Geometry check sheet. Reference: the model listing, model coordinates, mm. A direction names the side the tool comes from. Coordinates: 2 decimals unless noted, no trailing zeros. Order: outer loops, then holes, each group sorted by start corner. A loop starts at its lowest first (then second) coordinate and runs counter-clockwise, first axis right, second up. Notation, with made-up numbers: (23, 58.5) - (77, 58.5) arc R4 ccw to (77, 65.5) - close; hole circle Ø9 at (25, 61). An arc over 180 degrees is marked (long way). Put each result on its own line as item: value.
from build123d import *

# Parameters (mm, degrees)
SKETCH1_W                             = 152.4
SKETCH1_H                             = 203.2
BASE_DEPTH                            = 6.35
SKETCH2_W                             = 76.2
SKETCH2_H                             = 6.35
MOUNT_WALLS_DEPTH                     = 50.8
MOUNT_SUPPORT_DEPTH                   = 4.7625
F_24_0_152_DIAMETER_HOLE1_D           = 3.8608
F_24_0_152_DIAMETER_HOLE1_CSINK_D     = 5.1308
F_24_0_152_DIAMETER_HOLE1_CSINK_ANGLE = 90
SKETCH6_R                             = 8.89
SKETCH6_R_2                           = 1.55
CUT_EXTRUDE1_DEPTH                    = 149.785256326
SKETCH7_R                             = 10.16
SKETCH7_R_2                           = 1.55
CUT_EXTRUDE2_DEPTH                    = 6.35
CUT_EXTRUDE3_REACH                    = 138.783
SKETCH8_W                             = 38.1
SKETCH8_H                             = 101.6


with BuildPart() as part:
    # Sketch1 → base (new body)
    with BuildSketch(Plane.XY):
        Rectangle(SKETCH1_W, SKETCH1_H)
    extrude(amount=BASE_DEPTH)

    # Sketch2 → mount walls (add)
    with BuildSketch(Plane.XY.offset(6.35)):
        with Locations((38.1, -9.525)):
            Rectangle(SKETCH2_W, SKETCH2_H)
        with Locations((38.1, -60.325)):
            Rectangle(SKETCH2_W, SKETCH2_H)
    extrude(amount=MOUNT_WALLS_DEPTH)

    # Sketch3 → mount support (add)
    with BuildSketch(Plane(origin=(76.2, 0, 0), x_dir=(0, 0, -1), z_dir=(1, 0, 0))):
        Polygon((-6.35, -88.9), (-57.15, -63.5), (-6.35, -63.5), align=None)
        Polygon((-57.15, -6.35), (-6.35, 19.05), (-6.35, -6.35), align=None)
    mount_support = extrude(amount=-MOUNT_SUPPORT_DEPTH)

    # Mirror1: mount support across plane
    add(mount_support.mirror(Plane(origin=(38.1, 0, 0), x_dir=(0, 0, 1), z_dir=(1, 0, 0))))

    # #24 (0.152) Diameter Hole1 (through all)
    with Locations(Plane.XY.offset(6.35)):
        with Locations((-66.675, -92.075), (-66.675, 43.307), (-23.241, 43.307), (-23.241, -92.075), (-67.6275, 68.707), (-22.2885, 68.707)):
            CounterSinkHole(F_24_0_152_DIAMETER_HOLE1_D / 2, F_24_0_152_DIAMETER_HOLE1_CSINK_D / 2, counter_sink_angle=F_24_0_152_DIAMETER_HOLE1_CSINK_ANGLE)

    # Sketch6 → Cut-Extrude1 (cut, through all)
    with BuildSketch(Plane.XZ.offset(12.7)):
        with Locations((38.1, 38.1)):
            Circle(SKETCH6_R)
        with Locations((38.1, 50.62855)):
            Circle(SKETCH6_R_2)
        with Locations((38.1, 25.57145)):
            Circle(SKETCH6_R_2)
    extrude(amount=-CUT_EXTRUDE1_DEPTH, mode=Mode.SUBTRACT)

    # Sketch7 → Cut-Extrude2 (cut)
    with BuildSketch(Plane(origin=(0, -57.15, 0), x_dir=(1, 0, 0), z_dir=(0, 1, 0))):
        with Locations(Location((38.1, -38.1, 0), (0, 0, 180))):
            Circle(SKETCH7_R)
        with Locations(Location((24.2576, -46.091913366, 0), (0, 0, 180))):
            Circle(SKETCH7_R_2)
        with Locations(Location((38.1, -22.116173268, 0), (0, 0, 180))):
            Circle(SKETCH7_R_2)
        with Locations(Location((51.9424, -46.091913366, 0), (0, 0, 180))):
            Circle(SKETCH7_R_2)
    extrude(amount=-CUT_EXTRUDE2_DEPTH, mode=Mode.SUBTRACT)

    # Sketch8 → Cut-Extrude3 (cut, up to next)
    with BuildSketch(Plane.XY.offset(6.35), mode=Mode.PRIVATE) as cut_extrude3_sk1:
        Polygon((76.2, 42.338114892), (-35.744340046, 101.6), (76.2, 101.6), align=None)
    cut_extrude3_tool1 = extrude(cut_extrude3_sk1.sketch, amount=-CUT_EXTRUDE3_REACH, mode=Mode.PRIVATE) & part.part
    # Sketch8 → Cut-Extrude3 (cut, up to next)
    with BuildSketch(Plane.XY.offset(6.35), mode=Mode.PRIVATE) as cut_extrude3_sk2:
        with Locations((-44.31191896, -19.722477487)):
            Rectangle(SKETCH8_W, SKETCH8_H)
    cut_extrude3_tool2 = extrude(cut_extrude3_sk2.sketch, amount=-CUT_EXTRUDE3_REACH, mode=Mode.PRIVATE) & part.part
    add(cut_extrude3_tool1.solids().sort_by_distance((38.88522, 81.846038, 6.35))[0], mode=Mode.SUBTRACT)
    add(cut_extrude3_tool2.solids().sort_by_distance((-44.311919, -19.722477, 6.35))[0], mode=Mode.SUBTRACT)


solid = part.part
Q1. Thickness scan on L1, parallel to Z at x = 38, y = -60; L2, parallel to X at y = 5.5, z = 12.5; L3, parallel to Y at x = 43, z = 50.5. Record the ranges inside material, lowest first. Write a range as [from, to].
Answer block:
L1: z = [0, 20.57], [23.66, 27.94], [48.26, 57.15]
L2: x = [0, 4.76], [71.44, 76.2]
L3: y = [-63.5, -57.15], [-12.7, -6.35]
Q2. Section check B-B on y = -52. Record the boundary of the cut face in (x, z), then the cut area to 3 significant figures.
Answer block:
outline: (-76.2, 0) - (-63.36, 0) - (-63.36, 6.35) - (-76.2, 6.35) - close; (-25.26, 0) - (76.2, 0) - (76.2, 6.35) - (-25.26, 6.35) - close
area: 726 mm^2
Q3. Draft check along Y on faces 1 (the flat face through (-1, -101.6, 3)), 2 (the flat face through (-1, 1, 0)), 3 (the flat face through (29, -12.7, 31)), 4 (the flat face through (2.35, 6.17, 32.11)). Enter one of: pulls with the +Y half, pulls with the -Y half, needs draft (parallel to the pull), parting line crosses it, or undercut.
Answer block:
face 1: pulls with the -Y half
face 2: needs draft
face 3: undercut
face 4: pulls with the +Y half
Q4. Section check D-D on y = 8. Record the boundary of the cut face in (x, z), then the cut area to 3 significant figures.
Answer block:
outline: (-76.2, 0) - (-63.36, 0) - (-63.36, 6.35) - (-76.2, 6.35) - close; (-25.26, 0) - (76.2, 0) - (76.2, 28.45) - (71.44, 28.45) - (71.44, 6.35) - (4.76, 6.35) - (4.76, 28.45) - (0, 28.45) - (0, 6.35) - (-25.26, 6.35) - close
area: 936 mm^2
Q5. Depth check by flat-ended pin: pin 1 Ø3.5 at (x, z) = (24.26, 46.09) entering from -Y; pin 2 Ø4 at (x, z) = (38.1, 50.63) entering from +Y; pin 3 Ø10 at (x, y) = (10.5, -57) entering from +Z; pin 4 Ø6 at (x, y) = (-66.675, 43.307) entering from +Z. Enter the tip coordinate at first touch or a pass-through.
Answer block:
pin 1: stops at y = -63.5
pin 2: stops at y = -6.35
pin 3: stops at z = 57.15
pin 4: stops at z = 6.35
Q6. Section check C-C on z = 38.1. State how many separate pieces and enclosed holes the cut face has, then the cut area to 3 significant figures.
Answer block:
separate pieces: 4
enclosed holes: 0
area: 907 mm^2
Q7. Section check A-A on x = -50. Record the boundary of the cut face in (y, z).
Answer block:
outline: (-101.6, 0) - (-70.52, 0) - (-70.52, 6.35) - (-101.6, 6.35) - close; (31.08, 0) - (101.6, 0) - (101.6, 6.35) - (31.08, 6.35) - close
Q8. Access from +Z, -Z, +X, -X, +Y, -Y to the whole of each face (thin tool, end or side, straight path). Record for faces 5 (the cylindrical face through (33.412, -60.281, 29.086)), 6 (the flat face through (-45, 31.078, 3)), 7 (the flat face through (4.763, 1, 20)), 8 (the flat face through (38, -57.15, 26)).
Answer block:
face 5: -Y
face 6: +Z, -Z
face 7: +Z, +Y
face 8: +Z, +X, -X
